```python
from build123d import *

# Parameters (mm, degrees)
F0_W     = 6
F0_H     = 9.0617471188
F0_R     = 2
F1_DEPTH = 3
F2_D     = 3.5
F3_DEPTH = 15
F4_DEPTH = 6
F5_R     = 2.99999


# Not quite as in the source:
# - a fillet or chamfer is up to 0.001 mm smaller than in the source, because OpenCascade refuses the exact size
# - a feature names something its author has since deleted; it is built from what else it names


with BuildPart() as f1:
    # F0 (on Top) → F1 (new body)
    with BuildSketch(Plane.XY):
        Polygon((22.5, 5), (-22.5, 5), (-22.5, -5), (-16.5, -5), (16.5, -5), (22.5, -5), align=None)
        with Locations((-19.5, -9.5308735594)):
            Rectangle(F0_W, F0_H)
        with Locations((-19.5, -9)):
            Circle(F0_R, mode=Mode.SUBTRACT)
        with Locations((19.5, -9.5308735594)):
            Rectangle(F0_W, F0_H)
        with Locations((19.5, -9)):
            Circle(F0_R, mode=Mode.SUBTRACT)
        with Locations((-19.5, -9)):
            Circle(F0_R)
        with Locations((19.5, -9)):
            Circle(F0_R)
    extrude(amount=F1_DEPTH)

    # F2 (through all)
    with Locations(Plane(origin=(0, 0, 0), x_dir=(1, 0, 0), z_dir=(0, 0, -1))):
        with Locations((-17.5, 0), (17.5, 0)):
            Hole(F2_D / 2)

    # F0 (on Top) → F3 (join)
    with BuildSketch(Plane.XY):
        with Locations((-19.5, -9)):
            Circle(F0_R)
        with Locations((19.5, -9)):
            Circle(F0_R)
    extrude(amount=F3_DEPTH)

    # F0 (on Top) → F4 (join)
    with BuildSketch(Plane.XY):
        with Locations((-19.5, -9.5308735594)):
            Rectangle(F0_W, F0_H)
        with Locations((-19.5, -9)):
            Circle(F0_R, mode=Mode.SUBTRACT)
        with Locations((19.5, -9.5308735594)):
            Rectangle(F0_W, F0_H)
        with Locations((19.5, -9)):
            Circle(F0_R, mode=Mode.SUBTRACT)
        with Locations((-19.5, -9)):
            Circle(F0_R)
    extrude(amount=F4_DEPTH)

    # F5 (radius 3 in the source; OpenCascade refuses exactly that, so slightly less here)
    f5_edges = [f1.edges().sort_by_distance(p)[0] for p in [
        (-19.5, -5, 3),
        (19.5, -5, 3),
    ]]
    fillet(f5_edges, radius=F5_R)


solid = f1.part
```
Verification items for the finished model (mm, model axes). A direction names the side the tool comes from. Coordinates: 2 decimals unless noted, no trailing zeros. Order: outer loops, then holes, each group sorted by start corner. A loop starts at its lowest first (then second) coordinate and runs counter-clockwise, first axis right, second up. Notation, with made-up numbers: (-16.75, 9.5) - (26.25, 9.5) arc R23 cw to (26.25, 32.5) - close; hole circle Ø10 at (70, -14.75). An arc over 180 degrees is marked (long way). Return JSON: item names as keys, results as strings.
(1) Section check C-C, the plane y = 0. Record the cut outline in (x, z), and give its area (3 significant figures).
Filled sheet:
{"outline": "(-22.5, 0) - (-19.25, 0) - (-19.25, 3) - (-22.5, 3) - close; (-15.75, 0) - (15.75, 0) - (15.75, 3) - (-15.75, 3) - close; (19.25, 0) - (22.5, 0) - (22.5, 3) - (19.25, 3) - close", "area": "114 mm^2"}
(2) Mould release check, pull along X, two halves, no side actions. Record for faces 4 (the flat face through (22.5, -7, 2)), 5 (the flat face through (-22.5, -7, 2)), 6 (the flat face through (19.5, -11.5, 6)), 7 (the flat face through (0, 5, 1)): pulls with the +X half, pulls with the -X half, needs draft (parallel to the pull), parting line crosses it, or undercut.
Filled sheet:
{"face 4": "pulls with the +X half", "face 5": "pulls with the -X half", "face 6": "undercut", "face 7": "needs draft"}
(3) Go/stop test with flat-tipped pins: pin 1 (2.5 mm diameter, centred on x = 1.5, z = 1.5, fed in from -Y); pin 2 (6 mm diameter, centred on x = -5.5, y = 0, fed in from -Z); pin 3 (3 mm diameter, centred on y = -9.5, z = 8.5, fed in from -X); pin 4 (3 mm diameter, centred on x = 8.5, y = 1, fed in from +Z). Record where each tip stops, or that it passes through.
Filled sheet:
{"pin 1": "stops at y = -5", "pin 2": "stops at z = 0", "pin 3": "stops at x = -21.5", "pin 4": "stops at z = 3"}
(4) Section check D-D, the plane z = 4.25. Record the cut outline in (x, y).
Filled sheet:
{"outline": "(-22.5, -14.06) - (-16.5, -14.06) - (-16.5, -4.44) - (-22.5, -4.44) - close; (16.5, -14.06) - (22.5, -14.06) - (22.5, -4.44) - (16.5, -4.44) - close"}
(5) Section check A-A, the plane y = -12.5. Record the cut outline in (x, z).
Filled sheet:
{"outline": "(-22.5, 0) - (-16.5, 0) - (-16.5, 6) - (-22.5, 6) - close; (16.5, 0) - (22.5, 0) - (22.5, 6) - (16.5, 6) - close"}
(6) Section check B-B, the plane z = 1. Record the cut outline in (x, y).
Filled sheet:
{"outline": "(-22.5, -14.06) - (-16.5, -14.06) - (-16.5, -5) - (16.5, -5) - (16.5, -14.06) - (22.5, -14.06) - (22.5, 5) - (-22.5, 5) - close; hole circle Ø3.5 at (-17.5, 0); hole circle Ø3.5 at (17.5, 0)"}
(7) Thickness scan on line 1 along X through (y, z) = (-8.25, 3.25); line 2 along Y through (x, z) = (-17.5, 2.2); line 3 along Z through (x, y) = (2, 1.5). Record the ranges inside material, lowest first.
Filled sheet:
{"line 1": "x = -22.5 to -16.5, 16.5 to 22.5", "line 2": "y = -14.06 to -1.75, 1.75 to 5", "line 3": "z = 0 to 3"}
(8) Access from +Z, -Z, +X, -X, +Y, -Y to the whole of each face (thin tool, end or side, straight path). Record for faces 1 (the cylindrical face through (-20.974, -7.648, 10.437)), 2 (the flat face through (0, -5, 1)), 3 (the flat face through (0, 0, 3)).
Filled sheet:
{"face 1": "+Z", "face 2": "+Z, -Z, -Y", "face 3": "+Z, +Y"}
